```python
from build123d import *

# Parameters (mm, degrees)
SKETCH_R        = 47
SKETCH_R_2      = 45
PAD_DEPTH       = 15
PAD001_DEPTH    = 7
SKETCH002_R     = 18
POCKET_DEPTH    = 30.501
SKETCH003_R     = 5
SKETCH003_R_2   = 1.7
POCKET001_DEPTH = 22.001
SKETCH004_R     = 8.2
POCKET002_DEPTH = 9
SKETCH005_W     = 30.6
SKETCH005_H     = 7
POCKET003_DEPTH = 4
POCKET004_DEPTH = 7
POCKET005_DEPTH = 14
SKETCH008_R     = 2.6
POCKET006_DEPTH = 5


with BuildPart() as part:
    # Sketch → Pad (new body, symmetric)
    with BuildSketch(Plane.XY):
        Circle(SKETCH_R)
        Circle(SKETCH_R_2, mode=Mode.SUBTRACT)
    extrude(amount=PAD_DEPTH, both=True)

    # Sketch001 → Pad001 (join, symmetric)
    with BuildSketch(Plane.XY):
        with BuildLine():
            Line((-44.974993, 1.5), (-15, 1.5))
            Line((-15, 1.5), (-15, 11.5))
            ThreePointArc((-10, 16.5), (-13.535534, 15.035534), (-15, 11.5))
            Line((-10, 16.5), (10, 16.5))
            ThreePointArc((15, 11.5), (13.535534, 15.035534), (10, 16.5))
            Line((15, 11.5), (15, 1.5))
            Line((15, 1.5), (44.974993, 1.5))
            ThreePointArc((44.974993, -1.5), (45, 0), (44.974993, 1.5))
            Line((15, -1.5), (44.974993, -1.5))
            Line((15, -11.5), (15, -1.5))
            ThreePointArc((10, -16.5), (13.535534, -15.035534), (15, -11.5))
            Line((-10, -16.5), (10, -16.5))
            ThreePointArc((-15, -11.5), (-13.535534, -15.035534), (-10, -16.5))
            Line((-15, -1.5), (-15, -11.5))
            Line((-44.974993, -1.5), (-15, -1.5))
            ThreePointArc((-44.974993, 1.5), (-45, 0), (-44.974993, -1.5))
        make_face()
    extrude(amount=PAD001_DEPTH, both=True)

    # Sketch002 (on Face18 of Pad001) → Pocket (cut, through all)
    with BuildSketch(Plane.XZ.offset(16.5)):
        Circle(SKETCH002_R)
    extrude(amount=POCKET_DEPTH, mode=Mode.SUBTRACT)

    # Sketch003 (on Face7 of Pocket) → Pocket001 (cut, through all)
    with BuildSketch(Plane(origin=(0, 0, -7), x_dir=(1, 0, 0), z_dir=(0, 0, -1))):
        Circle(SKETCH003_R)
        with Locations((-11, 0)):
            Circle(SKETCH003_R_2)
        with Locations((11, 0)):
            Circle(SKETCH003_R_2)
    extrude(amount=-POCKET001_DEPTH, mode=Mode.SUBTRACT)

    # Sketch004 (on Face7 of Pocket001) → Pocket002 (cut)
    with BuildSketch(Plane(origin=(0, 0, -7), x_dir=(1, 0, 0), z_dir=(0, 0, -1))):
        Circle(SKETCH004_R)
    extrude(amount=-POCKET002_DEPTH, mode=Mode.SUBTRACT)

    # Sketch005 (on Face7 of Pocket002) → Pocket003 (cut)
    with BuildSketch(Plane(origin=(0, 0, -7), x_dir=(1, 0, 0), z_dir=(0, 0, -1))):
        Rectangle(SKETCH005_W, SKETCH005_H)
    extrude(amount=-POCKET003_DEPTH, mode=Mode.SUBTRACT)

    # Sketch006 (on Face9 of Pocket003) → Pocket004 (cut)
    with BuildSketch(Plane.XY.offset(7)):
        Polygon((-8.098815, -1.675), (-8.098815, 1.675), (-11, 3.35), (-13.901185, 1.675), (-13.901185, -1.675), (-11, -3.35), align=None)
        Polygon((11, -3.35), (13.901185, -1.675), (13.901185, 1.675), (11, 3.35), (8.098815, 1.675), (8.098815, -1.675), align=None)
    extrude(amount=-POCKET004_DEPTH, mode=Mode.SUBTRACT)

    # Sketch007 → Pocket005 (cut)
    with BuildSketch(Plane.XZ):
        Polygon((2.5, 4.330127), (-2.5, 4.330127), (-5, 0), (-2.5, -4.330127), (2.5, -4.330127), (5, 0), align=None)
    extrude(amount=POCKET005_DEPTH, mode=Mode.SUBTRACT)

    # Sketch008 (on Face23 of Pocket005) → Pocket006 (cut)
    with BuildSketch(Plane.XZ.offset(16.5)):
        Circle(SKETCH008_R)
    extrude(amount=-POCKET006_DEPTH, mode=Mode.SUBTRACT)


solid = part.part
```
Check sheet for the modelled part. Datum: model origin and axes. Units: mm. A direction names the side the tool comes from. Round coordinates to 2 decimals unless told otherwise and drop trailing zeros. Write each loop counter-clockwise with the first axis right and the second up, starting at its lowest first coordinate (ties: lowest second). Pieces come first, ordered by that corner, then holes. Notation, with made-up numbers: (-26.75, -36.75) -> (-0.75, -36.75) arc R14 ccw to (-0.75, -11.75) -> close; hole circle Ø8 at (-37, 28). An arc over 180 degrees is marked (long way). One line per question, with ' | ' between items. Start each with the question number.
1. Scan lines: line 1 along Y through (x, z) = (0, 5); line 2 along Y through (x, z) = (0, -4); line 3 along X through (y, z) = (0, -1). Record each from-to range of solid material in increasing order. Write a range as from..to.
2. Sectioned sample at B-B, the plane y = 23.5. Record the cut outline in (x, z), then the cut area to 3 significant figures.
3. Set-up check for faces 3 (the face through (18, -43, 0)), 4 (the face through (0, 6, 2)), 5 (the face through (-8.099, 0, 4)): record each of +Z, -Z, +X, -X, +Y, -Y from which the full face is reachable in a straight line by a thin tool's end or side.
4. Depth check by flat-ended pin: pin 1 (11 mm diameter, centred on x = 36.5, z = -1, fed in from -Y); pin 2 (4.5 mm diameter, centred on x = 10, y = 1, fed in from +Z); pin 3 (4 mm diameter, centred on x = -6, y = 10, fed in from -Z). Enter the tip coordinate at first touch or a pass-through.
5. Sectioned sample at A-A, the plane x = 0. Record the cut outline in (y, z), then the cut area to 3 significant figures.
6. Release check for a two-part mould opening along X. For faces 1 (the face through (17, 42, 15)), 2 (the face through (-30, -1.5, 0)) record: +X half, -X half, draft (parallel to the pull), parting line (faces both ways), or undercut.
7. Sectioned sample at C-C, the plane x = 25.5. Record the cut outline in (y, z).
8. Sectioned sample at D-D, the plane y = -26. Record the cut outline in (x, z), then the cut area to 3 significant figures.
Taken from the geometry:
1) line 1: y = -16.5..-5, 5..16.5, 45..47 | line 2: y = -16.5..-14, 8.2..16.5, 45..47 | line 3: x = -47..-12.7, -9.3..-8.2, 8.2..9.3, 12.7..47
2) outline: (-40.7, -15) -> (-38.38, -15) -> (-38.38, 15) -> (-40.7, 15) -> close; (38.38, -15) -> (40.7, -15) -> (40.7, 15) -> (38.38, 15) -> close | area: 140 mm^2
3) face 3: -Y | face 4: -Z | face 5: +Z
4) pin 1: stops at y = -35.33 | pin 2: stops at z = 7 | pin 3: stops at z = -7
5) outline: (-16.5, -7) -> (-8.2, -7) -> (-8.2, -4.33) -> (-14, -4.33) -> (-14, -2.6) -> (-16.5, -2.6) -> close; (-16.5, 2.6) -> (-14, 2.6) -> (-14, 4.33) -> (-5, 4.33) -> (-5, 7) -> (-16.5, 7) -> close; (5, 2) -> (8.2, 2) -> (8.2, -7) -> (16.5, -7) -> (16.5, 7) -> (5, 7) -> close; (45, -15) -> (47, -15) -> (47, 15) -> (45, 15) -> close | area: 254 mm^2
6) face 1: draft | face 2: undercut
7) outline: (-39.48, -15) -> (-37.08, -15) -> (-37.08, 15) -> (-39.48, 15) -> close; (-1.5, -7) -> (1.5, -7) -> (1.5, 7) -> (-1.5, 7) -> close; (37.08, -15) -> (39.48, -15) -> (39.48, 15) -> (37.08, 15) -> close
8) outline: (-39.15, -15) -> (-36.73, -15) -> (-36.73, 15) -> (-39.15, 15) -> close; (36.73, -15) -> (39.15, -15) -> (39.15, 15) -> (36.73, 15) -> close | area: 145 mm^2
